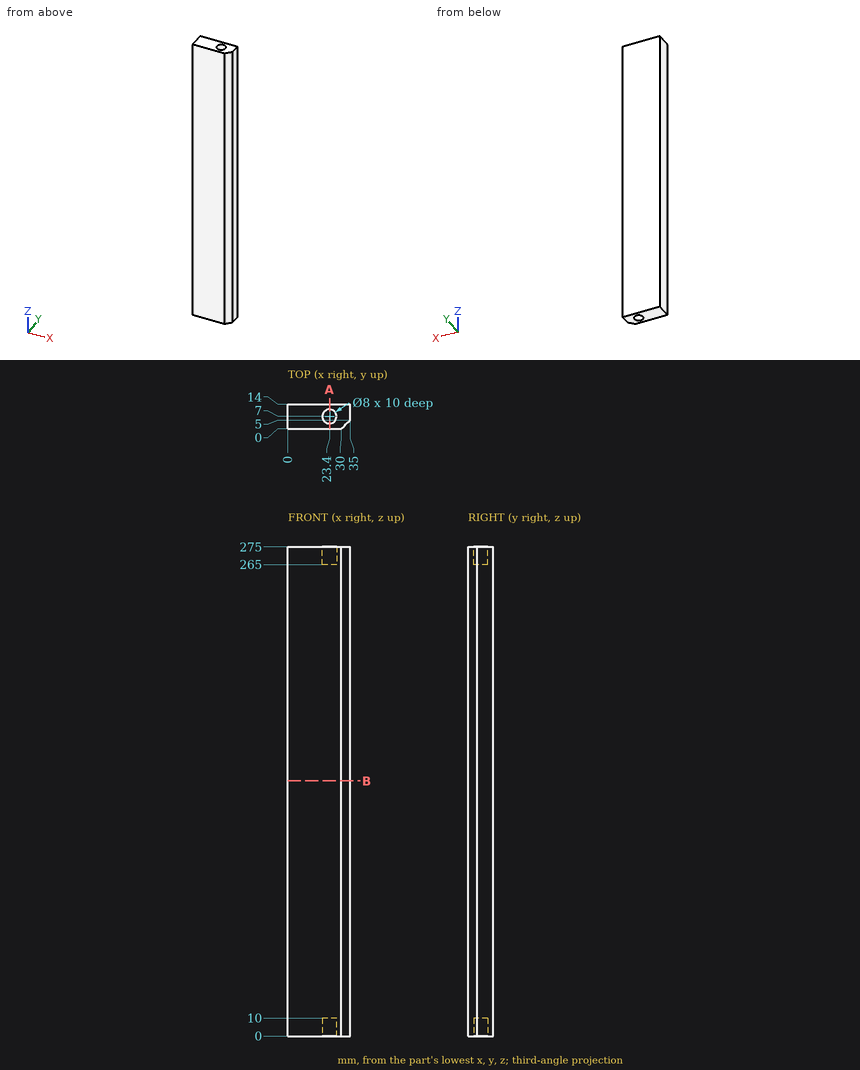
Study the drawing (mm; zero at the part's minimum x, y, z) and answer. Give positions to 0.01 mm unless a question says otherwise; leave off trailing zeros. Order: outer loops, then holes, each group sorted by start corner. A loop starts at its lowest first (then second) coordinate and runs counter-clockwise, first axis right, second up.
1) Consider line 1 along Y through (x, z) = (23.4, 7); line 2 along X through (y, z) = (2.5, 151). Determine where each line is inside the solid, lowest interval first.
Reported:
line 1: y = 0 to 3, 11 to 14
line 2: x = 0 to 32.5
2) Find section A-A on x = 23.4. Write down the section's boundary in (y, z).
Reported:
outline: (0, 0) - (3, 0) - (3, 10) - (11, 10) - (11, 0) - (14, 0) - (14, 275) - (11, 275) - (11, 265) - (3, 265) - (3, 275) - (0, 275) - close
3) Find section B-B on z = 143.5. Write down the section's boundary in (x, y), then the cut area to 4 significant figures.
Reported:
outline: (0, 0) - (30, 0) - (35, 5) - (35, 14) - (0, 14) - close
area: 477.5 mm2
4) Given P1, Ø8, axis at y = 4, z = 151.5, coming from the +X side; P2, Ø7, axis at x = 23.4, y = 7, coming from the -Z side; P3, Ø4, axis at x = 23.5, y = 8, coming from the +Z side, each flat-ended and moving along its own axis, determine where each tip first touches the part or whether it passes through.
Reported:
P1: stops at x = 35
P2: stops at z = 10
P3: stops at z = 265
